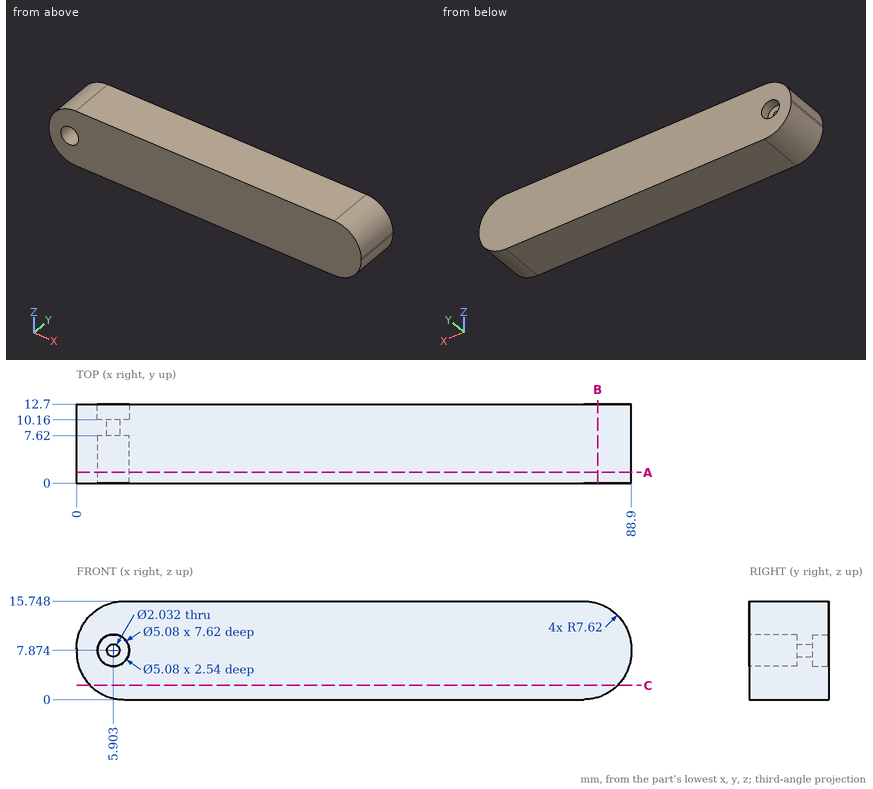
Here's the drawing with two shaded views (mm, measured from the low corner). I have some questions. Coordinates: 2 decimals unless noted, no trailing zeros. Write each loop counter-clockwise with the first axis right and the second up, starting at its lowest first coordinate (ties: lowest second). Pieces come first, ordered by that corner, then holes.
Item 1: I want a section at A-A on y = 1.75. Write out the boundary of the cut face in (x, z).
Item 2: I want a section at C-C on z = 2.25. Write out the boundary of the cut face in (x, y).
Item 3: Will these pins go through, and if not, where does the flat tip stop? pin 1 (1.5 mm diameter, centred on x = 6, z = 8.5, fed in from +Y); pin 2 (6 mm diameter, centred on y = 9, z = 3, fed in from +X); pin 3 (1.2 mm diameter, centred on x = 5.9, z = 7.87, fed in from -Y); pin 4 (1.5 mm diameter, centred on x = 6, z = 6.5, fed in from -Y).
Item 4: I want a section at B-B on x = 83.5. Write out the boundary of the cut face in (y, z).
Item 5: If I drill on line 1 (X direction, y = 1, z = 8.25) (1 decimal); line 2 (X direction, y = 11.5, z = 6) (1 decimal); line 3 (Z direction, x = 6.5, y = 12) (1 decimal), over which ranges is the centre line in solid material (lowest first)?
Findings below:
1. outline: (0, 7.62) arc R7.62 ccw to (7.62, 0) - (81.28, 0) arc R7.62 ccw to (88.9, 7.62) - (88.9, 8.13) arc R7.62 ccw to (81.28, 15.75) - (7.62, 15.75) arc R7.62 ccw to (0, 8.13) - close; hole circle Ø5.08 at (5.9, 7.87)
2. outline: (2.21, 0) - (86.69, 0) - (86.69, 12.7) - (2.21, 12.7) - close
3. pin 1: stops at y = 10.16
3. pin 2: stops at x = 88.73
3. pin 3: passes through
3. pin 4: stops at y = 7.62
4. outline: (0, 0.33) - (12.7, 0.33) - (12.7, 15.42) - (0, 15.42) - close
5. line 1: x = 0 to 3.4, 8.4 to 88.9
5. line 2: x = 0.2 to 4.2, 7.6 to 88.7
5. line 3: z = 0.1 to 5.4, 10.3 to 15.7
